The figure shows three views and two pictorial views of one solid part (mm, origin at its lowest corner). Answer the questions. A direction names the side the tool comes from. Coordinates: 2 decimals unless noted, no trailing zeros. Write each loop counter-clockwise with the first axis right and the second up, starting at its lowest first coordinate (ties: lowest second). Pieces come first, ordered by that corner, then holes.
Item 1: Section B-B (z = 5.75) is taken. Give the vertices of the cut face in (x, y).
Item 2: Determine the mould class of the marked faces 3, 4 and 5 for opening direction X: released by +X, released by -X, zero draft, split by the parting line, or undercut.
Item 3: A tool of negligible diameter and unlimited length cuts with its end or side. For the marked faces 1 and 2, from which of +Z, -Z, +X, -X, +Y, -Y can it reach the whole face along a straight path? Write none if from no direction.
Item 4: Each of these flat-tipped pins is pushed along its axis until it touches: P1, Ø2.5, axis at x = 3.5, z = 5.5, coming from the +Y side; P2, Ø1, axis at x = 4.5, y = 1, coming from the +Z side (1 decimal); P3, Ø0.5, axis at y = 1, z = 4, coming from the +X side. Where does it stop, or does it pass through?
Item 5: Section C-C (y = 1) is taken. Give the vertices of the cut face in (x, z) (1 decimal), then the cut area to 3 significant figures.
Item 6: Section D-D (z = 7.75) is taken. Give the vertices of the cut face in (x, y).
Item 7: Straight lines are drawn through the part: probe 1 along Y at (x, z) = (1.5, 5.5); probe 2 along Z at (x, y) = (3.25, 1) (1 decimal); probe 3 along X at (y, z) = (1.6, 5.5). For each, find the intervals that lie inside material, in ascending order.
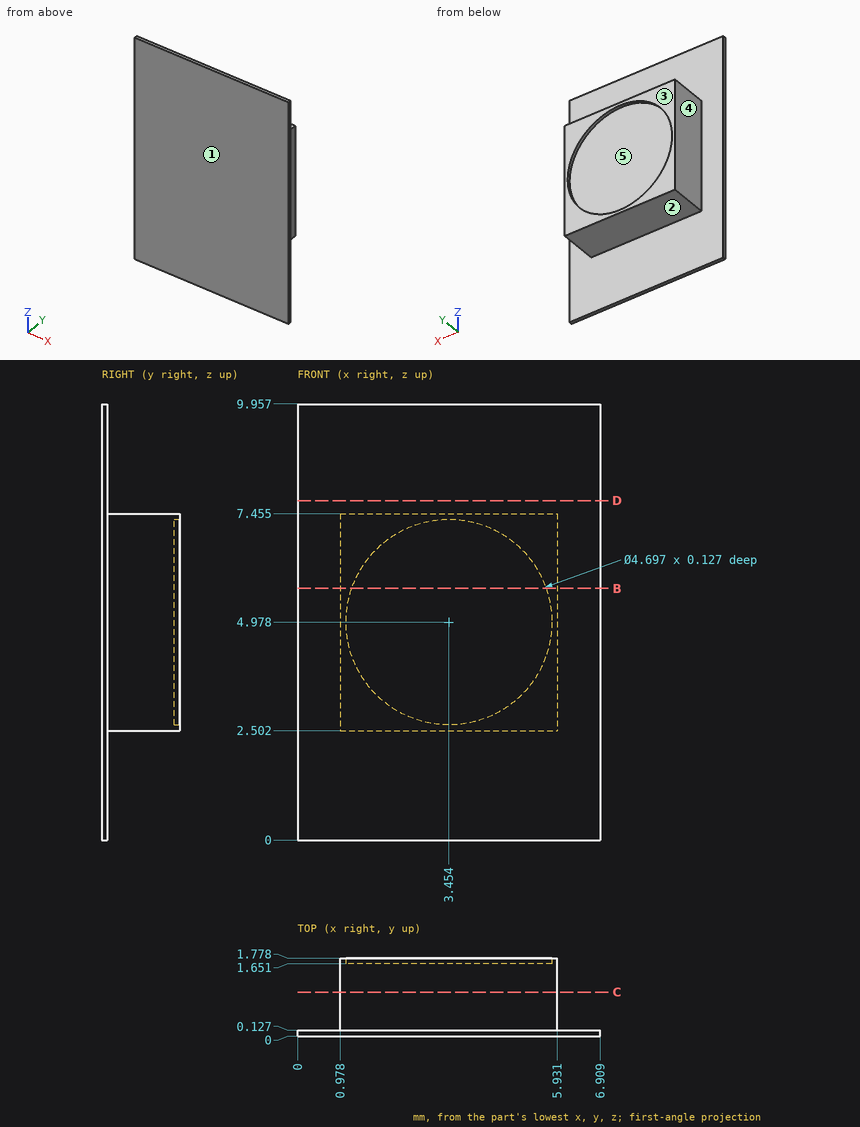
Established:
1. outline: (0, 0) - (6.91, 0) - (6.91, 0.13) - (5.93, 0.13) - (5.93, 1.78) - (5.67, 1.78) - (5.67, 1.65) - (1.24, 1.65) - (1.24, 1.78) - (0.98, 1.78) - (0.98, 0.13) - (0, 0.13) - close
2. face 3: zero draft
2. face 4: released by -X
2. face 5: undercut
3. face 1: +Z, -Z, +X, -X, -Y
3. face 2: -Z, +X, -X, +Y
4. P1: stops at y = 1.65
4. P2: stops at z = 7.5
4. P3: stops at x = 5.93
5. outline: (1, 2.5) - (5.9, 2.5) - (5.9, 7.5) - (1, 7.5) - close
5. area: 24.5 mm2
6. outline: (0, 0) - (6.91, 0) - (6.91, 0.13) - (0, 0.13) - close
7. probe 1: y = 0 to 1.65
7. probe 2: z = 2.5 to 7.5
7. probe 3: x = 0.98 to 5.93
